Model file for the job. Use its own axes, mm. Round coordinates to 2 decimals unless told otherwise and drop trailing zeros. Order: outer loops, then holes, each group sorted by start corner. A loop starts at its lowest first (then second) coordinate and runs counter-clockwise, first axis right, second up. Notation, with made-up numbers: (8.5, 71.5) - (13.5, 71.5) arc R20 cw to (13.5, 86.5) - close; hole circle Ø11 at (-15, 14). An arc over 180 degrees is marked (long way). Put each result on its own line as item: value. Start each with the question number.
Item 1: Saw through at B-B on y = 268.5. List the corners of the cut face in (x, z), plus the area to 3 significant figures.
Item 2: Pin check, flat tips, straight feed: pin 1 Ø1.5 at (y, z) = (56, 3.5) entering from +X; pin 2 Ø2.5 at (x, z) = (88.5, 3) entering from +Y; pin 3 Ø1.5 at (y, z) = (126, 2) entering from -X. Stop position of each tip, or through.
Item 3: Saw through at A-A on z = 1.5. State how many separate pieces and enclosed holes the cut face has, plus the area to 3 significant figures.
Item 4: Probe probe 1 along Y at (x, z) = (32.5, 1.15); probe 2 along X at (y, z) = (116, 2.05). List the from-to ranges inside material, lowest first.
```python
from build123d import *

# Parameters (mm, degrees)
SKETCH1_W           = 180
SKETCH1_H           = 300
SKETCH1_R           = 2.25
BOSS_EXTRUDE1_DEPTH = 5
CUT_EXTRUDE1_REACH  = 315.249
SKETCH2_W           = 5
SKETCH2_H           = 37.5


with BuildPart() as part:
    # Sketch1 → Boss-Extrude1 (new body)
    with BuildSketch(Plane.XY):
        with Locations((0, 150)):
            Rectangle(SKETCH1_W, SKETCH1_H)
        with Locations((-32.5, 150)):
            Circle(SKETCH1_R, mode=Mode.SUBTRACT)
        with Locations((32.5, 150)):
            Circle(SKETCH1_R, mode=Mode.SUBTRACT)
    extrude(amount=BOSS_EXTRUDE1_DEPTH)

    # Sketch2 → Cut-Extrude1 (cut, up to next)
    with BuildSketch(Plane.XY.offset(5), mode=Mode.PRIVATE) as cut_extrude1_sk1:
        with Locations((-87.5, 281.25)):
            Rectangle(SKETCH2_W, SKETCH2_H)
    cut_extrude1_tool1 = extrude(cut_extrude1_sk1.sketch, amount=-CUT_EXTRUDE1_REACH, mode=Mode.PRIVATE) & part.part
    # Sketch2 → Cut-Extrude1 (cut, up to next)
    with BuildSketch(Plane.XY.offset(5), mode=Mode.PRIVATE) as cut_extrude1_sk2:
        with Locations((-87.5, 206.25)):
            Rectangle(SKETCH2_W, SKETCH2_H)
    cut_extrude1_tool2 = extrude(cut_extrude1_sk2.sketch, amount=-CUT_EXTRUDE1_REACH, mode=Mode.PRIVATE) & part.part
    # Sketch2 → Cut-Extrude1 (cut, up to next)
    with BuildSketch(Plane.XY.offset(5), mode=Mode.PRIVATE) as cut_extrude1_sk3:
        with Locations((-87.5, 131.25)):
            Rectangle(SKETCH2_W, SKETCH2_H)
    cut_extrude1_tool3 = extrude(cut_extrude1_sk3.sketch, amount=-CUT_EXTRUDE1_REACH, mode=Mode.PRIVATE) & part.part
    # Sketch2 → Cut-Extrude1 (cut, up to next)
    with BuildSketch(Plane.XY.offset(5), mode=Mode.PRIVATE) as cut_extrude1_sk4:
        with Locations((-87.5, 56.25)):
            Rectangle(SKETCH2_W, SKETCH2_H)
    cut_extrude1_tool4 = extrude(cut_extrude1_sk4.sketch, amount=-CUT_EXTRUDE1_REACH, mode=Mode.PRIVATE) & part.part
    # Sketch2 → Cut-Extrude1 (cut, up to next)
    with BuildSketch(Plane.XY.offset(5), mode=Mode.PRIVATE) as cut_extrude1_sk5:
        with Locations((87.5, 281.25)):
            Rectangle(SKETCH2_W, SKETCH2_H)
    cut_extrude1_tool5 = extrude(cut_extrude1_sk5.sketch, amount=-CUT_EXTRUDE1_REACH, mode=Mode.PRIVATE) & part.part
    # Sketch2 → Cut-Extrude1 (cut, up to next)
    with BuildSketch(Plane.XY.offset(5), mode=Mode.PRIVATE) as cut_extrude1_sk6:
        with Locations((87.5, 206.25)):
            Rectangle(SKETCH2_W, SKETCH2_H)
    cut_extrude1_tool6 = extrude(cut_extrude1_sk6.sketch, amount=-CUT_EXTRUDE1_REACH, mode=Mode.PRIVATE) & part.part
    # Sketch2 → Cut-Extrude1 (cut, up to next)
    with BuildSketch(Plane.XY.offset(5), mode=Mode.PRIVATE) as cut_extrude1_sk7:
        with Locations((87.5, 131.25)):
            Rectangle(SKETCH2_W, SKETCH2_H)
    cut_extrude1_tool7 = extrude(cut_extrude1_sk7.sketch, amount=-CUT_EXTRUDE1_REACH, mode=Mode.PRIVATE) & part.part
    # Sketch2 → Cut-Extrude1 (cut, up to next)
    with BuildSketch(Plane.XY.offset(5), mode=Mode.PRIVATE) as cut_extrude1_sk8:
        with Locations((87.5, 56.25)):
            Rectangle(SKETCH2_W, SKETCH2_H)
    cut_extrude1_tool8 = extrude(cut_extrude1_sk8.sketch, amount=-CUT_EXTRUDE1_REACH, mode=Mode.PRIVATE) & part.part
    add(cut_extrude1_tool1.solids().sort_by_distance((-87.5, 281.25, 5))[0], mode=Mode.SUBTRACT)
    add(cut_extrude1_tool2.solids().sort_by_distance((-87.5, 206.25, 5))[0], mode=Mode.SUBTRACT)
    add(cut_extrude1_tool3.solids().sort_by_distance((-87.5, 131.25, 5))[0], mode=Mode.SUBTRACT)
    add(cut_extrude1_tool4.solids().sort_by_distance((-87.5, 56.25, 5))[0], mode=Mode.SUBTRACT)
    add(cut_extrude1_tool5.solids().sort_by_distance((87.5, 281.25, 5))[0], mode=Mode.SUBTRACT)
    add(cut_extrude1_tool6.solids().sort_by_distance((87.5, 206.25, 5))[0], mode=Mode.SUBTRACT)
    add(cut_extrude1_tool7.solids().sort_by_distance((87.5, 131.25, 5))[0], mode=Mode.SUBTRACT)
    add(cut_extrude1_tool8.solids().sort_by_distance((87.5, 56.25, 5))[0], mode=Mode.SUBTRACT)


solid = part.part
```
Results found:
1. outline: (-85, 0) - (85, 0) - (85, 5) - (-85, 5) - close
1. area: 850 mm²
2. pin 1: stops at x = 85
2. pin 2: stops at y = 262.5
2. pin 3: stops at x = -85
3. separate pieces: 1
3. enclosed holes: 2
3. area: 52,500 mm²
4. probe 1: y = 0 to 147.75, 152.25 to 300
4. probe 2: x = -85 to 85
